Study the drawing (mm; zero at the part's minimum x, y, z) and answer. A direction names the side the tool comes from. Round coordinates to 2 decimals unless told otherwise and drop trailing zeros. Write each loop counter-clockwise with the first axis right and the second up, starting at its lowest first coordinate (ties: lowest second). Pieces come first, ordered by that corner, then holes. Notation, with made-up numbers: (47, -6.75) - (103, -6.75) arc R12 ccw to (103, 2.25) - close; hole circle Ø11 at (-29, 89). An arc over 180 degrees is marked (long way). Return JSON: item names as keys, results as strings. Group by question number.
(1) Section A-A, the plane z = 6.75 is taken. Write down the section's boundary in (x, y).
(2) Find the intervals of material crossed by line 1 along Z through (x, y) = (16.5, 21); line 2 along X through (y, z) = (2.75, 3.5), in increasing order. Write a range as [from, to].
(3) Section B-B, the plane y = 11 is taken. Write down the section's boundary in (x, z).
(4) Each of these flat-tipped pins is pushed along its axis until it touches: pin 1 (5 mm diameter, centred on x = 41, z = 13.5, fed in from -Y); pin 2 (12.5 mm diameter, centred on x = 31, y = 16.5, fed in from -Z); pin 3 (3 mm diameter, centred on y = 11, z = 12, fed in from +X). Where does it stop, or does it pass through?
(5) Which of the six approach directions +Z, -Z, +X, -X, +Y, -Y give full straight-line access (tool end or side, diameter ignored) to the marked faces 1 and 2?
(6) Section C-C, the plane x = 54 is taken. Write down the section's boundary in (y, z), then the cut area to 3 significant figures.
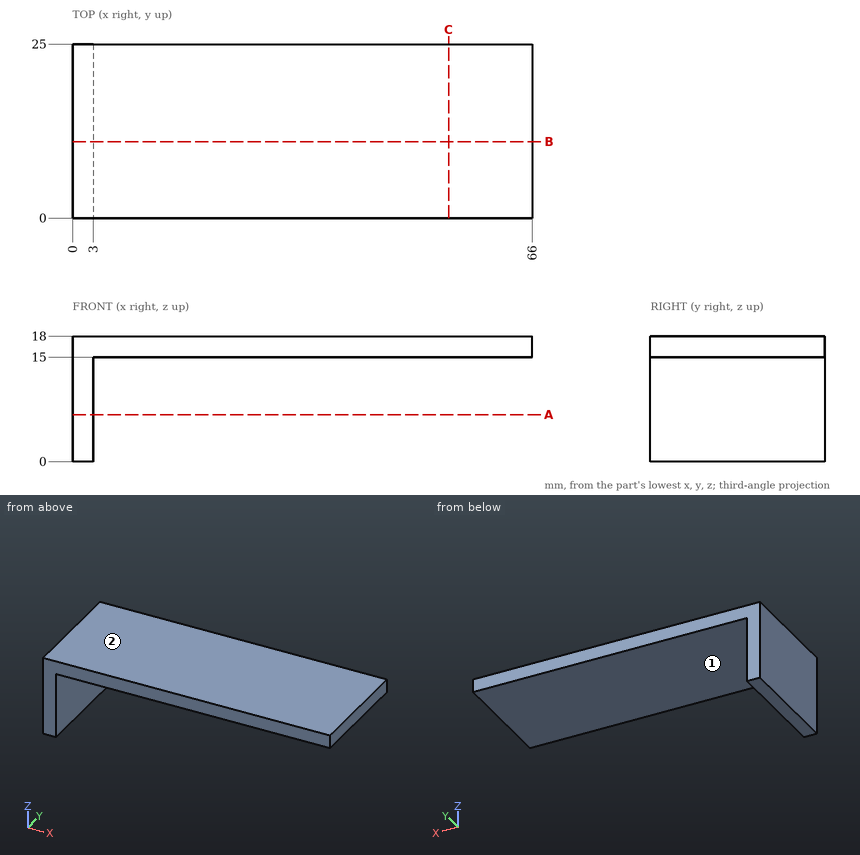
Working result:
{
 "1": {"outline": "(0, 0) - (3, 0) - (3, 25) - (0, 25) - close"},
 "2": {"line 1": "z = [15, 18]", "line 2": "x = [0, 3]"},
 "3": {"outline": "(0, 0) - (3, 0) - (3, 15) - (66, 15) - (66, 18) - (0, 18) - close"},
 "4": {"pin 1": "stops at y = 0", "pin 2": "stops at z = 15", "pin 3": "stops at x = 3"},
 "5": {"face 1": "-Z, +X, +Y, -Y", "face 2": "+Z, +X, -X, +Y, -Y"},
 "6": {"outline": "(0, 15) - (25, 15) - (25, 18) - (0, 18) - close", "area": "75.0 mm^2"}
}
